Job drawing, mm, ordinate dimensions from the low corner. One solid piece. A direction names the side the tool comes from. Give positions to 0.01 mm unless a question says otherwise; leave off trailing zeros. Order: outer loops, then holes, each group sorted by start corner. A loop starts at its lowest first (then second) coordinate and runs counter-clockwise, first axis right, second up.
1. Which spindle directions (+Z, -Z, +X, -X, +Y, -Y) get a long thin tool onto all of the face, cutting with end or side? Do the marked faces 1 and 2. Say none if no direction does.
2. Slice it at D-D on x = 27.5. List the corners of the cut face in (y, z) (1 decimal), and give its area (3 significant figures).
3. Probe line 1 (Y direction, x = 26, z = 23); line 2 (Z direction, x = 27, y = 6.25) (1 decimal); line 3 (X direction, y = 3.25, z = 13) (1 decimal). List the from-to ranges inside material, lowest first.
4. Drop flat-ended pins along their axis: pin 1 Ø2 at (x, y) = (12.5, 10) entering from +Z (3 decimals); pin 2 Ø5 at (x, z) = (24, 22) entering from -Y. Give the stop position or say it passes through.
5. Slice it at B-B on z = 4.5. List the corners of the cut face in (x, y).
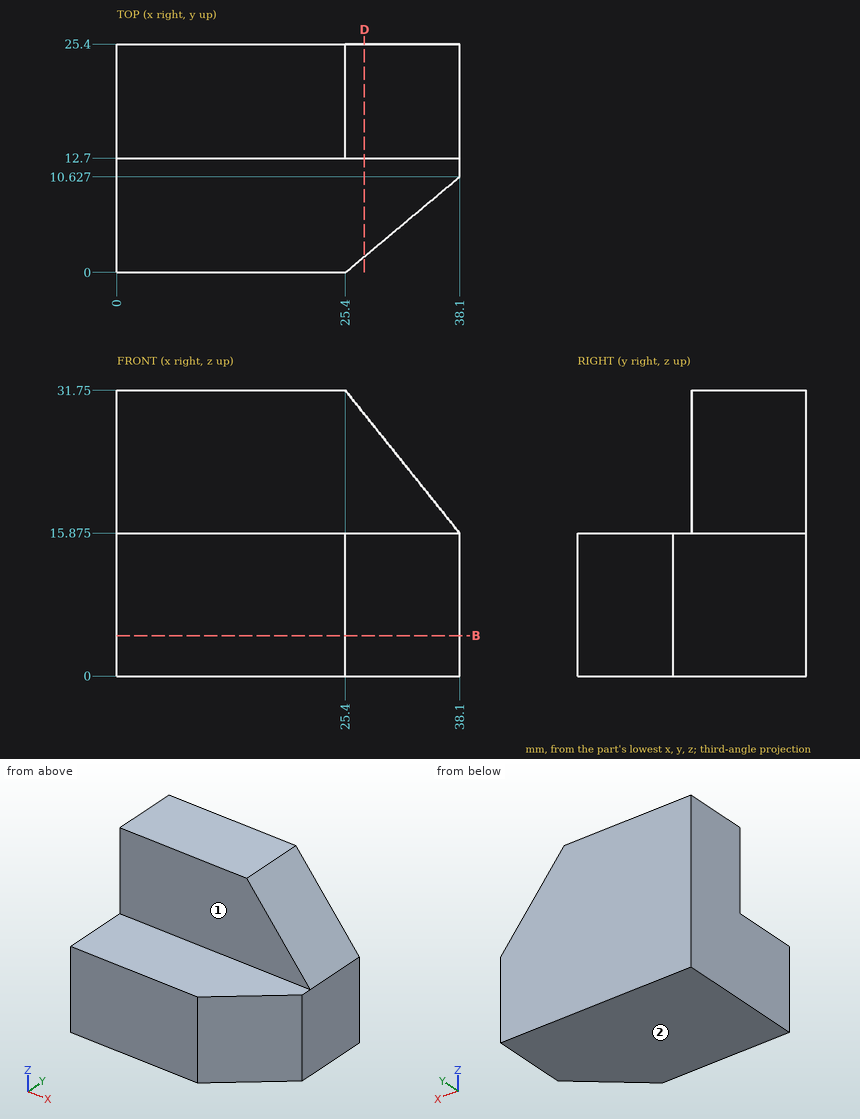
Data:
1. face 1: +Z, +X, -X, -Y
1. face 2: -Z, +X, -X, +Y, -Y
2. outline: (1.8, 0) - (25.4, 0) - (25.4, 29.1) - (12.7, 29.1) - (12.7, 15.9) - (1.8, 15.9) - close
2. area: 544 mm2
3. line 1: y = 12.7 to 25.4
3. line 2: z = 0 to 15.9
3. line 3: x = 0 to 29.3
4. pin 1: stops at z = 15.875
4. pin 2: stops at y = 12.7
5. outline: (0, 0) - (25.4, 0) - (38.1, 10.63) - (38.1, 25.4) - (0, 25.4) - close
